```python
from build123d import *

# Parameters (mm, degrees)
F2_DEPTH  = 19.05
F3_W      = 254
F3_H      = 50.8
F4_DEPTH  = 152.4
F5_W      = 19.05
F5_H      = 152.4
F6_DEPTH  = 107.95
F7_R      = 63.5
F8_DEPTH  = 127
F9_R      = 44.45
F10_DEPTH = 146.051


# Not quite as in the source:
# - a variable given as a bare number and used for a length is read in inches; the dataset says mm whatever the document's units were


with BuildPart() as f2:
    # F1 (on Front) → F2 (new body)
    with BuildSketch(Plane.XZ):
        with BuildLine():
            Line((-254, 0), (0, 0))
            Line((0, 0), (0, 50.8))
            Line((0, 50.8), (-67.7722531834, 226.0981223472))
            ThreePointArc((-67.7722531834, 226.0981223472), (-127, 266.7), (-186.2277468166, 226.0981223472))
            Line((-186.2277468166, 226.0981223472), (-254, 50.8))
            Line((-254, 50.8), (-254, 0))
        make_face()
    extrude(amount=F2_DEPTH)

    # F3 (on face) → F4 (join)
    with BuildSketch(Plane.XZ.offset(19.05)):
        with Locations((-127, 25.4)):
            Rectangle(F3_W, F3_H)
    extrude(amount=F4_DEPTH)

    # F5 (on face) → F6 (join)
    with BuildSketch(Plane.XZ.offset(19.05)):
        with Locations((-127, 127)):
            Rectangle(F5_W, F5_H)
    extrude(amount=F6_DEPTH)

    # F7 (on face) → F8 (join)
    with BuildSketch(Plane.XZ.offset(19.05)):
        with Locations((-127, 203.2)):
            Circle(F7_R)
    extrude(amount=F8_DEPTH)

    # F9 (on face) → F10 (cut, through all)
    with BuildSketch(Plane.XZ.offset(146.05)):
        with Locations((-127, 203.2)):
            Circle(F9_R)
    extrude(amount=-F10_DEPTH, mode=Mode.SUBTRACT)


solid = f2.part
```
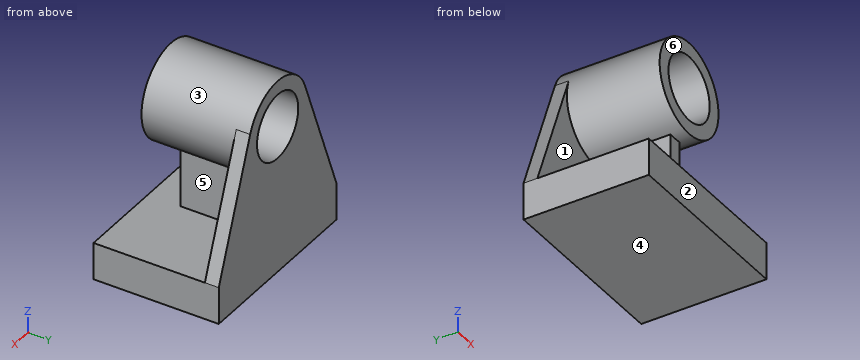
Check sheet for the modelled part. Datum: model origin and axes. Units: mm. Face numbers are marked on the shaded views. A direction names the side the tool comes from. Round coordinates to 2 decimals unless told otherwise and drop trailing zeros. Write each loop counter-clockwise with the first axis right and the second up, starting at its lowest first coordinate (ties: lowest second). Pieces come first, ordered by that corner, then holes. Notation, with made-up numbers: (22, 24.5) -> (42, 24.5) arc R12 ccw to (42, 36.5) -> close; hole circle Ø11 at (16.5, 24). An arc over 180 degrees is marked (long way). Put each result on its own line as item: value.
(1) Tool access check on the marked faces 1, 2 and 3. Record the directions out of +Z, -Z, +X, -X, +Y, -Y that give a thin tool (end or side, any length) a straight path to the whole face; none if there is none.
Values found:
face 1: -X, -Y
face 2: +Z, -Z, +X, -X, -Y
face 3: -Y
(2) Sectioned sample at B-B (y = -40). Enter the section's corners in (x, z) (3 decimals).
Values found:
outline: (-254, 0) -> (0, 0) -> (0, 50.8) -> (-117.475, 50.8) -> (-117.475, 140.418) arc R63.5 ccw (long way) to (-136.525, 140.418) -> (-136.525, 50.8) -> (-254, 50.8) -> close; hole circle Ø88.9 at (-127, 203.2)
(3) Go/stop test with flat-tipped pins: pin 1 Ø5 at (y, z) = (-144, 225.5) entering from -X; pin 2 Ø8 at (y, z) = (-123, 101) entering from -X (3 decimals); pin 3 Ø1.5 at (x, z) = (-167, 222) entering from -Y. Record where each tip stops, or that it passes through.
Values found:
pin 1: stops at x = -187.33
pin 2: stops at x = -136.525
pin 3: stops at y = -146.05
(4) Sectioned sample at D-D (y = -155). Enter the section's corners in (x, z).
Values found:
outline: (-254, 0) -> (0, 0) -> (0, 50.8) -> (-254, 50.8) -> close
(5) Mould release check, pull along Z, two halves, no side actions. Record for the marked faces 4, 5 and 6: released by +Z, released by -Z, zero draft, split by the parting line, or undercut.
Values found:
face 4: released by -Z
face 5: undercut
face 6: zero draft
(6) Sectioned sample at C-C (z = 203.2). Enter the section's corners in (x, y), plus the area to 3 significant figures.
Values found:
outline: (-195.08, -19.05) -> (-190.5, -19.05) -> (-190.5, -146.05) -> (-171.45, -146.05) -> (-171.45, 0) -> (-195.08, 0) -> close; (-82.55, -146.05) -> (-63.5, -146.05) -> (-63.5, -19.05) -> (-58.92, -19.05) -> (-58.92, 0) -> (-82.55, 0) -> close
area: 5,740 mm^2
(7) Material ranges on line 1 (Z direction, x = -127, y = -87); line 2 (X direction, y = -53, z = 203); line 3 (Z direction, x = -90.5, y = -42), recorded low to high.
Values found:
line 1: z = 0 to 158.75, 247.65 to 266.7
line 2: x = -190.5 to -171.45, -82.55 to -63.5
line 3: z = 0 to 50.8, 151.24 to 177.83, 228.57 to 255.16
(8) Sectioned sample at A-A (x = -127). Enter the section's corners in (y, z).
Values found:
outline: (-171.45, 0) -> (0, 0) -> (0, 158.75) -> (-146.05, 158.75) -> (-146.05, 139.7) -> (-127, 139.7) -> (-127, 50.8) -> (-171.45, 50.8) -> close; (-146.05, 247.65) -> (0, 247.65) -> (0, 266.7) -> (-146.05, 266.7) -> close
